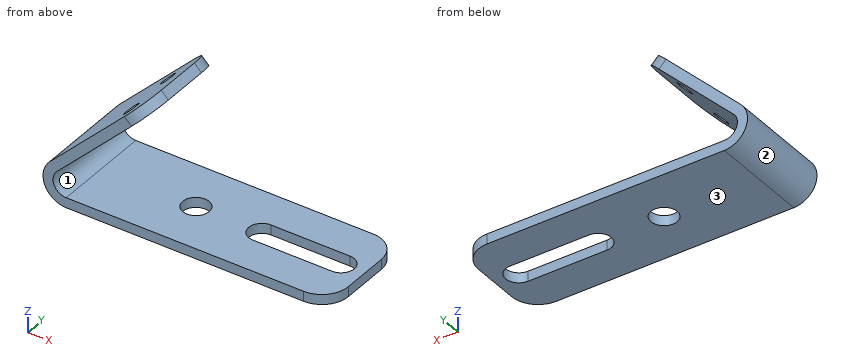
```python
from build123d import *

# Parameters (mm, degrees)
F1_DEPTH = 241.935
F2_R     = 63.5
F3_DEPTH = 48.261
F4_R     = 127
F5_R     = 127
F6_R     = 38.1
F7_DEPTH = 76.2


with BuildPart() as f1:
    # F0 (on Front) → F1 (new body, symmetric)
    with BuildSketch(Plane.XZ):
        with BuildLine():
            Line((369.986552, 528.03906), (-79.026254, 79.026254))
            ThreePointArc((-79.026254, 79.026254), (-103.252777, -42.7687), (0, -111.76))
            Line((0, -111.76), (1270, -111.76))
            Line((1270, -111.76), (1270, -63.5))
            Line((1270, -63.5), (0, -63.5))
            ThreePointArc((0, -63.5), (-58.66635, -24.300398), (-44.901281, 44.901281))
            Line((-44.901281, 44.901281), (404.111525, 493.914087))
            Line((404.111525, 493.914087), (369.986552, 528.03906))
        make_face()
    extrude(amount=F1_DEPTH, both=True)

    # F2 (on face) → F3 (cut, through all)
    with BuildSketch(Plane.XY.offset(-63.5)):
        with Locations((457.2, 0)):
            Circle(F2_R)
        with BuildLine():
            Line((1155.7, 63.5), (774.7, 63.5))
            ThreePointArc((774.7, 63.5), (711.2, 0), (774.7, -63.5))
            Line((774.7, -63.5), (1155.7, -63.5))
            ThreePointArc((1155.7, -63.5), (1219.2, 0), (1155.7, 63.5))
        make_face()
    extrude(amount=-F3_DEPTH, mode=Mode.SUBTRACT)

    # F4
    f4_edges = [f1.edges().sort_by_distance(p)[0] for p in [
        (1270, -241.935, -87.63),
        (1270, 241.935, -87.63),
    ]]
    fillet(f4_edges, radius=F4_R)

    # F5
    f5_edges = [f1.edges().sort_by_distance(p)[0] for p in [
        (387.049039, -241.935, 510.976573),
        (387.049039, 241.935, 510.976573),
    ]]
    fillet(f5_edges, radius=F5_R)

    # F6 (on face) → F7 (cut)
    with BuildSketch(Plane(origin=(-79.026254, 0, 79.026254), x_dir=(0, -1, 0), z_dir=(-0.707107, 0, 0.707107))):
        with Locations((-127.635, 444.5)):
            Circle(F6_R)
        with Locations((127.635, 444.5)):
            Circle(F6_R)
    extrude(amount=-F7_DEPTH, mode=Mode.SUBTRACT)


solid = f1.part
```
The model under review builds one solid part; all positions refer to its coordinate system, in mm. Face numbers are marked on the shaded views. Round coordinates to 2 decimals unless told otherwise and drop trailing zeros. Loops run counter-clockwise (first coordinate to the right, second up) from the corner with the lowest first, then second, coordinate; pieces in that order, holes last. Notation, with made-up numbers: (-34, -13.5) -> (10, -13.5) arc R30 cw to (10, 25.5) -> close; hole circle Ø10 at (-39, 1). An arc over 180 degrees is marked (long way). Answer as a JSON object with one key per item and string values. Group by question number.
1) For pin 1 Ø4 at (y, z) = (133, 170) entering from -X; pin 2 Ø6 at (x, y) = (420, -94.5) entering from +Z; pin 3 Ø5 at (y, z) = (-36, 181.5) entering from -X, all flat-tipped, find the tip position at first contact; note any pin that passes through.
2) We need section C-C on x = 645.5. Write out the cut boundary in (y, z) (3 decimals).
3) Mouldability with a two-part tool opening along Z and no side actions: class the marked faces 1, 2 and 3 as released by +Z, released by -Z, zero draft, split by the parting line, or undercut.
4) We need section A-A on y = 0. Write out the cut boundary in (x, z), then the cut area to 3 significant figures.
5) For line 1 (X direction, y = -24.5, z = -84); line 2 (Y direction, x = 457, z = -92) (3 decimals); line 3 (Z direction, x = 446, y = 177), list the stretches that pass through material, from the lowest coordinate up. Write a range as [from, to].
6) We need section B-B on x = 457.2. Write out the cut boundary in (y, z) (3 decimals), then the cut area to 3 significant figures.
7) We need section D-D on y = 212. Write out the cut boundary in (x, z), then the cut area to 3 significant figures.
Result set:
{
 "1": {"pin 1": "x = 9.95", "pin 2": "z = -63.5", "pin 3": "x = 20.95"},
 "2": {"outline": "(-241.935, -111.76) -> (241.935, -111.76) -> (241.935, -63.5) -> (-241.935, -63.5) -> close"},
 "3": {"face 1": "undercut", "face 2": "split by the parting line", "face 3": "released by -Z"},
 "4": {"outline": "(-79.03, 79.03) arc R111.76 ccw to (0, -111.76) -> (393.7, -111.76) -> (393.7, -63.5) -> (0, -63.5) arc R63.5 cw to (-44.9, 44.9) -> (404.11, 493.91) -> (369.99, 528.04) -> close; (520.7, -111.76) -> (711.2, -111.76) -> (711.2, -63.5) -> (520.7, -63.5) -> close; (1219.2, -111.76) -> (1270, -111.76) -> (1270, -63.5) -> (1219.2, -63.5) -> close", "area": "71,300 mm²"},
 "5": {"line 1": "[-73.72, 398.62], [515.78, 716.12], [1214.28, 1270]", "line 2": "[-241.935, -63.5], [63.5, 241.935]", "line 3": "[-111.76, -63.5]"},
 "6": {"outline": "(-241.935, -111.76) -> (-63.5, -111.76) -> (-63.5, -63.5) -> (-241.935, -63.5) -> close; (63.5, -111.76) -> (241.935, -111.76) -> (241.935, -63.5) -> (63.5, -63.5) -> close", "area": "17,200 mm²"},
 "7": {"outline": "(-79.03, 79.03) arc R111.76 ccw to (0, -111.76) -> (1224.9, -111.76) -> (1224.9, -63.5) -> (0, -63.5) arc R63.5 cw to (-44.9, 44.9) -> (372.22, 462.02) -> (338.1, 496.15) -> close", "area": "97,500 mm²"}
}
